Work out the finished part from the listing and answer in its coordinate system (mm). A direction names the side the tool comes from. Round coordinates to 2 decimals unless told otherwise and drop trailing zeros. Write each loop counter-clockwise with the first axis right and the second up, starting at its lowest first coordinate (ties: lowest second). Pieces come first, ordered by that corner, then holes. Notation, with made-up numbers: M 89,26.5 L 93,26.5 A18 ccw 93,60.5 Z; hole C 23,72.25 d4. An arc over 180 degrees is marked long. One line per item, written item: value. Start each with the question number.
Q1. Find section D-D (y = 9). Write down the section's boundary in (x, z) (3 decimals).
Q2. Find section C-C (z = -21). Count the separate pieces of the cut face and the enclosed holes in it, and give its area (3 significant figures).
Q3. The mould has two halves that part along Z. Classify faces 4 (the flat face through (36, -13.945, -7)), 5 (the flat face through (33, -14.945, -14)), 6 (the flat face through (-3, 5, -28)), 7 (the cylindrical face through (-32.89, -14.44, -19.99)): released by +Z, released by -Z, zero draft, split by the parting line, or undercut.
Q4. Given pin 1 Ø1 at (y, z) = (6, -5.5) entering from -X; pin 2 Ø4 at (x, z) = (34, -7) entering from +Y; pin 3 Ø4 at (x, z) = (35, -21) entering from +Y, each flat-ended and moving along its own axis, determine where each tip first touches the part or whether it passes through.
Q5. Consider probe 1 along Z at (x, y) = (-34, -12.65); probe 2 along Z at (x, y) = (34, -14.7); probe 3 along X at (y, z) = (-12.5, -11) (3 decimals). Determine where each line is inside the solid, lowest interval first.
Q6. A tool of negligible diameter and unlimited length cuts with its end or side. For faces 1 (the flat face through (-29.875, -8, -14)), 2 (the cylindrical face through (33.46, -12.93, -4.56)), 3 (the flat face through (-31.125, -6, -14)), from which of +Z, -Z, +X, -X, +Y, -Y can it reach the whole face along a straight path? Write none if from no direction.
Q7. Find section B-B (x = 34). Write down the section's boundary in (y, z), and give its area (3 significant figures).
Q8. Find section A-A (y = -4). Write down the section's boundary in (x, z) (3 decimals), and give its area (3 significant figures).
from build123d import *

# Parameters (mm, degrees)
SALIENTE_EXTRUIR1_DEPTH = 28
CROQUIS2_R              = 2.5
CROQUIS2_R_2            = 1.5
CROQUIS2_R_3            = 1.407949101
CORTAR_EXTRUIR1_DEPTH   = 2
CROQUIS3_R              = 1.407949101
CROQUIS3_R_2            = 1.5
CORTAR_EXTRUIR2_DEPTH   = 54.570618198
CROQUIS4_R              = 1.407949101
CROQUIS4_R_2            = 1.5
CORTAR_EXTRUIR3_DEPTH   = 54.570618198


with BuildPart() as part:
    # Croquis1 → Saliente-Extruir1 (new body)
    with BuildSketch(Plane.XY):
        with BuildLine():
            ThreePointArc((-29.875, 0), (-16.125, 13.75), (-2.375, 0))
            Line((-2.375, 0), (-1.125, 0))
            Line((-1.125, 0), (1.125, 0))
            Line((1.125, 0), (2.375, 0))
            ThreePointArc((2.375, 0), (16.125, 13.75), (29.875, 0))
            Line((29.875, 0), (29.875, -9.945231658))
            Line((29.875, -9.945231658), (29.875, -14.945231658))
            Line((29.875, -14.945231658), (36.875, -14.945231658))
            Line((36.875, -14.945231658), (36.875, -11.945231658))
            Line((36.875, -11.945231658), (31.125, -11.945231658))
            Line((31.125, -11.945231658), (31.125, 0))
            ThreePointArc((31.125, 0), (17.63263443, 14.924042295), (1.428061543, 3))
            Line((1.428061543, 3), (-1.428061543, 3))
            ThreePointArc((-1.428061543, 3), (-17.63263443, 14.924042295), (-31.125, 0))
            Line((-31.125, 0), (-31.125, -11.945231658))
            Line((-31.125, -11.945231658), (-36.875, -11.945231658))
            Line((-36.875, -11.945231658), (-36.875, -14.945231658))
            Line((-36.875, -14.945231658), (-29.875, -14.945231658))
            Line((-29.875, -14.945231658), (-29.875, -9.945231658))
            Line((-29.875, -9.945231658), (-29.875, 0))
        make_face()
    extrude(amount=-SALIENTE_EXTRUIR1_DEPTH)

    # Croquis2 → Cortar-Extruir1 (cut)
    # profile 1 of 4: a face of its own
    with BuildSketch(Plane(origin=(0, -11.945231658, 0), x_dir=(1, 0, 0), z_dir=(0, 1, 0))):
        with Locations(Location((-34, 21, 0), (0, 0, 180))):
            Circle(CROQUIS2_R)
        with Locations(Location((-34, 21, 0), (0, 0, 180))):
            Circle(CROQUIS2_R_2, mode=Mode.SUBTRACT)
    # profile 2 of 4: a face of its own
    with BuildSketch(Plane(origin=(0, -11.945231658, 0), x_dir=(1, 0, 0), z_dir=(0, 1, 0))):
        with Locations(Location((-34, 7, 0), (0, 0, 180))):
            Circle(CROQUIS2_R)
        with Locations(Location((-34, 7, 0), (0, 0, 180))):
            Circle(CROQUIS2_R_3, mode=Mode.SUBTRACT)
    # profile 3 of 4: a face of its own
    with BuildSketch(Plane(origin=(0, -11.945231658, 0), x_dir=(1, 0, 0), z_dir=(0, 1, 0))):
        with Locations((34, 7)):
            Circle(CROQUIS2_R)
        with Locations((34, 7)):
            Circle(CROQUIS2_R_3, mode=Mode.SUBTRACT)
    # profile 4 of 4: a face of its own
    with BuildSketch(Plane(origin=(0, -11.945231658, 0), x_dir=(1, 0, 0), z_dir=(0, 1, 0))):
        with Locations((34, 21)):
            Circle(CROQUIS2_R)
        with Locations((34, 21)):
            Circle(CROQUIS2_R_2, mode=Mode.SUBTRACT)
    extrude(amount=-CORTAR_EXTRUIR1_DEPTH, mode=Mode.SUBTRACT)

    # Croquis3 → Cortar-Extruir2 (cut, through all)
    with BuildSketch(Plane(origin=(0, -11.945231658, 0), x_dir=(1, 0, 0), z_dir=(0, 1, 0))):
        with Locations(Location((-34, 7, 0), (0, 0, 180))):
            Circle(CROQUIS3_R)
        with Locations(Location((-34, 21, 0), (0, 0, 180))):
            Circle(CROQUIS3_R_2)
    extrude(amount=-CORTAR_EXTRUIR2_DEPTH, mode=Mode.SUBTRACT)

    # Croquis4 → Cortar-Extruir3 (cut, through all)
    with BuildSketch(Plane(origin=(0, -11.945231658, 0), x_dir=(1, 0, 0), z_dir=(0, 1, 0))):
        with Locations(Location((34, 7, 0), (0, 0, 180))):
            Circle(CROQUIS4_R)
        with Locations(Location((34, 21, 0), (0, 0, 180))):
            Circle(CROQUIS4_R_2)
    extrude(amount=-CORTAR_EXTRUIR3_DEPTH, mode=Mode.SUBTRACT)


solid = part.part
The answers:
1. outline: M -28.125,-28 L -26.52,-28 L -26.52,0 L -28.125,0 Z; M -5.73,-28 L -4.125,-28 L -4.125,0 L -5.73,0 Z; M 4.125,-28 L 5.73,-28 L 5.73,0 L 4.125,0 Z; M 26.52,-28 L 28.125,-28 L 28.125,0 L 26.52,0 Z
2. separate pieces: 3
2. enclosed holes: 0
2. area: 166 mm2
3. face 4: undercut
3. face 5: zero draft
3. face 6: released by -Z
3. face 7: undercut
4. pin 1: x = -30.08
4. pin 2: y = -13.95
4. pin 3: y = -11.95
5. probe 1: -28 to -23.5, -18.5 to -9.5, -4.5 to 0
5. probe 2: -28 to -22.5, -19.5 to -8.41, -5.59 to 0
5. probe 3: -36.875 to -29.875, 29.875 to 36.875
6. face 1: +Z, -Z, -Y
6. face 2: +Y
6. face 3: +Z, -Z, -X, +Y
7. outline: M -14.95,-28 L -11.95,-28 L -11.95,-23.5 L -13.95,-23.5 L -13.95,-22.5 L -14.95,-22.5 Z; M -14.95,-19.5 L -13.95,-19.5 L -13.95,-18.5 L -11.95,-18.5 L -11.95,-9.5 L -13.95,-9.5 L -13.95,-8.41 L -14.95,-8.41 Z; M -14.95,-5.59 L -13.95,-5.59 L -13.95,-4.5 L -11.95,-4.5 L -11.95,0 L -14.95,0 Z
7. area: 58.2 mm2
8. outline: M -31.125,-28 L -29.875,-28 L -29.875,0 L -31.125,0 Z; M 29.875,-28 L 31.125,-28 L 31.125,0 L 29.875,0 Z
8. area: 70.0 mm2
